Geometry: final body of the model. Coordinates: model frame, mm. Face numbers are marked on the shaded views. A direction names the side the tool comes from. Coordinates: 2 decimals unless noted, no trailing zeros. Loops run counter-clockwise (first coordinate to the right, second up) from the corner with the lowest first, then second, coordinate; pieces in that order, holes last. Notation, with made-up numbers: (31.5, 70.25) - (58.5, 70.25) arc R27 ccw to (58.5, 97.25) - close; hole circle Ø1 at (-1, 85). An arc over 180 degrees is marked (long way). Put each result on its own line as item: value. Start each with the question number.
1) Draft query along X for the marked faces 1, 2, 3 and 4. Return one class per face: +X half, -X half, draft (parallel to the pull), parting line (faces both ways), or undercut.
2) Section A-A on z = 4.75. Output: boundary loops of the cut face in (x, y), and give its area (3 significant figures).
3) Section C-C on y = 2.5. Output: boundary loops of the cut face in (x, z), and give its area (3 significant figures).
4) Contact query for flat-ended pins moving along their axis: pin 1 Ø2.5 at (x, z) = (9, 7) entering from -Y; pin 2 Ø1 at (y, z) = (-3, 1) entering from -X; pin 3 Ø1.6 at (x, z) = (8.5, 1.5) entering from -Y. Output: stop coordinate, or through.
5) Material intervals for line 1 along Z through (x, y) = (8.5, 0.85); line 2 along X through (y, z) = (0.75, 10); line 3 along X through (y, z) = (3.9, 1.5), sorted ascending. Write a range as from..to.
6) Section D-D on y = -2.5. Output: boundary loops of the cut face in (x, z), and give its area (3 significant figures).
7) Section B-B on x = 8.5. Output: boundary loops of the cut face in (y, z), and give its area (3 significant figures).
8) Reachability of the marked faces 5 and 6 from +Z, -Z, +X, -X, +Y, -Y: full face, straight path, thin tool, end or side. Return the list, or none.
```python
from build123d import *
from build123d.topology import SkipClean

# Parameters (mm, degrees)
SKETCH_1_W          = 10
SKETCH_1_H          = 12
EXTRUDE_1_DEPTH     = 5
SKETCH_2_R          = 0.7
CUT_EXTRUDE_1_DEPTH = 17.401219467
SKETCH_2_3_R        = 3.25
CUT_EXTRUDE_2_DEPTH = 17.401219467
SKETCH_2_4_R        = 1
CUT_EXTRUDE_3_DEPTH = 3
EXTRUDE_START       = 3.9
EXTRUDE_2_DEPTH     = 3.9
SKETCH_4_R          = 0.35
CUT_EXTRUDE_4_DEPTH = 16.00833102


with BuildPart() as part:
    # 草图1 → 凸台-拉伸1 (new body)
    with BuildSketch(Plane(origin=(0, 0, 0), x_dir=(1, 0, 0), z_dir=(0, 1, 0))):
        with Locations((5, -6)):
            Rectangle(SKETCH_1_W, SKETCH_1_H)
    extrude(amount=EXTRUDE_1_DEPTH)

    # 草图2 → 切除-拉伸1 (cut, through all)
    with BuildSketch(Plane.XZ):
        with Locations(Location((1.5, 1.5, 0), (0, 0, 270))):
            Circle(SKETCH_2_R)
        with Locations(Location((1.5, 10.5, 0), (0, 0, 270))):
            Circle(SKETCH_2_R)
        with Locations(Location((8.5, 10.5, 0), (0, 0, 270))):
            Circle(SKETCH_2_R)
        with Locations(Location((8.5, 1.5, 0), (0, 0, 270))):
            Circle(SKETCH_2_R)
    extrude(amount=-CUT_EXTRUDE_1_DEPTH, mode=Mode.SUBTRACT)

    # 草图2<3> → 切除-拉伸2 (cut, through all)
    with BuildSketch(Plane.XZ):
        with Locations(Location((5, 6, 0), (0, 0, 270))):
            Circle(SKETCH_2_3_R)
    extrude(amount=-CUT_EXTRUDE_2_DEPTH, mode=Mode.SUBTRACT)

    # 草图2<4> → 切除-拉伸3 (cut)
    with BuildSketch(Plane.XZ):
        with Locations(Location((1.5, 10.5, 0), (0, 0, 270))):
            Circle(SKETCH_2_4_R)
        with Locations(Location((8.5, 10.5, 0), (0, 0, 270))):
            Circle(SKETCH_2_4_R)
        with Locations(Location((8.5, 1.5, 0), (0, 0, 270))):
            Circle(SKETCH_2_4_R)
        with Locations(Location((1.5, 1.5, 0), (0, 0, 270))):
            Circle(SKETCH_2_4_R)
    extrude(amount=-CUT_EXTRUDE_3_DEPTH, mode=Mode.SUBTRACT)

    # 草图3 → 凸台-拉伸2 (add)
    with SkipClean():  # the faces are left unmerged after this step: merging them gives an invalid solid
        with BuildSketch(Plane.XZ.offset(EXTRUDE_START)):
            with BuildLine():
                Line((2.5, 8.6), (3.05, 8.6))
                ThreePointArc((3.05, 8.6), (5, 9.25), (6.95, 8.6))
                Line((6.95, 8.6), (7.5, 8.6))
                Line((7.5, 8.6), (7.5, 12))
                Line((7.5, 12), (2.5, 12))
                Line((2.5, 12), (2.5, 8.6))
            make_face()
            with BuildLine():
                Line((2.5, 3.4), (2.5, 0))
                Line((2.5, 0), (7.5, 0))
                Line((7.5, 0), (7.5, 3.4))
                Line((7.5, 3.4), (6.95, 3.4))
                ThreePointArc((6.95, 3.4), (5, 2.75), (3.05, 3.4))
                Line((3.05, 3.4), (2.5, 3.4))
            make_face()
        extrude(amount=-EXTRUDE_2_DEPTH)

    # 草图4 → 切除-拉伸4 (cut, through all)
    with SkipClean():  # the faces are left unmerged after this step: merging them gives an invalid solid
        with BuildSketch(Plane.ZY.offset(-2.5)):
            with Locations((10.3, -1.95)):
                Circle(SKETCH_4_R)
            with Locations((1.7, -1.95)):
                Circle(SKETCH_4_R)
        extrude(amount=-CUT_EXTRUDE_4_DEPTH, mode=Mode.SUBTRACT)


solid = part.part
```
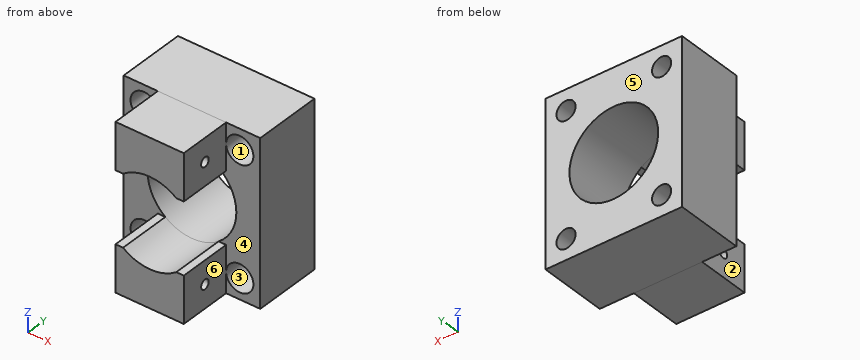
Answer block:
1. face 1: undercut
1. face 2: -X half
1. face 3: undercut
1. face 4: draft
2. outline: (0, 0) - (2, 0) - (2, 5) - (0, 5) - close; (8, 0) - (10, 0) - (10, 5) - (8, 5) - close
2. area: 20.0 mm²
3. outline: (0, 0) - (10, 0) - (10, 12) - (0, 12) - close; hole circle Ø2 at (1.5, 1.5); hole circle Ø2 at (1.5, 10.5); hole circle Ø6.5 at (5, 6); hole circle Ø2 at (8.5, 1.5); hole circle Ø2 at (8.5, 10.5)
3. area: 74.3 mm²
4. pin 1: stops at y = 0
4. pin 2: stops at x = 2.5
4. pin 3: stops at y = 3
5. line 1: z = 0..0.5, 2.5..9.5, 11.5..12
5. line 2: x = 0..0.63, 2.37..7.63, 9.37..10
5. line 3: x = 0..0.8, 2.2..7.8, 9.2..10
6. outline: (2.5, 0) - (7.5, 0) - (7.5, 3.4) - (6.95, 3.4) arc R3.25 cw to (3.05, 3.4) - (2.5, 3.4) - close; (2.5, 8.6) - (3.05, 8.6) arc R3.25 cw to (6.95, 8.6) - (7.5, 8.6) - (7.5, 12) - (2.5, 12) - close
6. area: 30.5 mm²
7. outline: (0, 0) - (5, 0) - (5, 0.8) - (3, 0.8) - (3, 0.5) - (0, 0.5) - close; (0, 2.5) - (3, 2.5) - (3, 2.2) - (5, 2.2) - (5, 9.8) - (3, 9.8) - (3, 9.5) - (0, 9.5) - close; (0, 11.5) - (3, 11.5) - (3, 11.2) - (5, 11.2) - (5, 12) - (0, 12) - close
7. area: 42.4 mm²
8. face 5: +Z, -Z, +X, -X, +Y
8. face 6: +Z, -Z, +X, -Y
